Input: part model. Units: mm. Frame: model coordinates. Round coordinates to 2 decimals unless told otherwise and drop trailing zeros. Write each question's results on one line, items separated by ' | '.
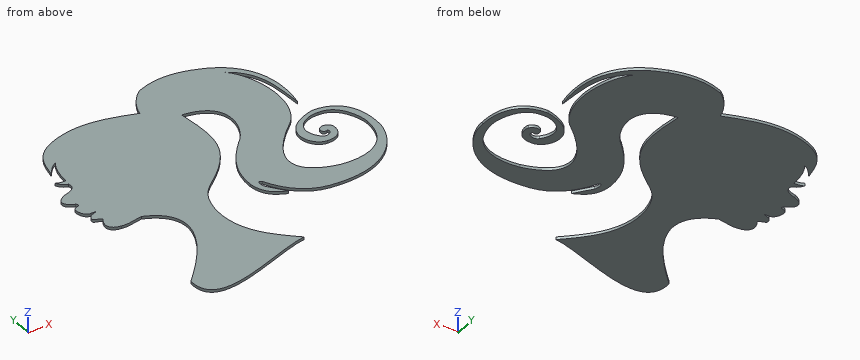
from build123d import *

# Parameters (mm, degrees)
F1_DEPTH = 1


with BuildPart() as f1:
    # F0 (on Top) → F1 (new body)
    with BuildSketch(Plane.XY):
        with BuildLine():
            add(Edge.make_bspline(
                [(-20.8665426716, 18.397650235), (-20.1903553635, 22.148523992), (-18.5927961308, 30.6072682277), (0.8297736088, 36.4578977579), (13.424566628, 32.0204028302), (19.7537988424, 29.7199543566)],
                knots=[0, 0, 0, 0, 0.276946376, 0.6257935478, 1, 1, 1, 1], degree=3))
            add(Edge.make_bspline(
                [(-20.8665426716, 18.397650235), (-19.5796533177, 19.9643534919), (-18.4618644416, 21.7904262245), (-16.4070501924, 22.4652308971)],
                knots=[0, 0, 0, 0, 6.0359163029, 6.0359163029, 6.0359163029, 6.0359163029], degree=3))
            add(Edge.make_bspline(
                [(-19.1014725715, 12.8793083131), (-19.1014725715, 16.4545979351), (-18.215386197, 20.5580331385), (-16.4070501924, 22.4652308971)],
                knots=[0, 0, 0, 0, 9.957400451, 9.957400451, 9.957400451, 9.957400451], degree=3))
            add(Edge.make_bspline(
                [(-22.681472823, 13.5721871629), (-21.7005256563, 12.9922945052), (-20.227715373, 12.7012068406), (-19.1014725715, 12.8793083131)],
                knots=[0, 0, 0, 0, 3.6464342722, 3.6464342722, 3.6464342722, 3.6464342722], degree=3))
            add(Edge.make_bspline(
                [(-19.5205342025, 10.8836535364), (-21.142622456, 11.263910681), (-22.0586042851, 12.5462869182), (-22.681472823, 13.5721871629)],
                knots=[0, 0, 0, 0, 4.1496681824, 4.1496681824, 4.1496681824, 4.1496681824], degree=3))
            add(Edge.make_bspline(
                [(-23.7308889627, 6.6631692462), (-21.9120476395, 7.1236696094), (-18.5412317514, 7.9297339544), (-19.5205342025, 10.8836535364)],
                knots=[0, 0, 0, 0, 5.9615077667, 5.9615077667, 5.9615077667, 5.9615077667], degree=3))
            add(Edge.make_bspline(
                [(-23.7308889627, 0.8257346926), (-26.2068863958, 1.7335914308), (-29.0413927287, 4.5064790174), (-23.7308889627, 6.6631692462)],
                knots=[0, 0, 0, 0, 5.8374345535, 5.8374345535, 5.8374345535, 5.8374345535], degree=3))
            add(Edge.make_bspline(
                [(-23.7308889627, -0.4696604155), (-23.3873687685, -0.4872174759), (-22.8560995311, 0.2822079114), (-23.7308889627, 0.8257346926)],
                knots=[0, 0, 0, 0, 1.2953951082, 1.2953951082, 1.2953951082, 1.2953951082], degree=3))
            add(Edge.make_bspline(
                [(-25.4408102483, -1.531884307), (-25.1299161464, -0.9100947645), (-24.4304016232, -0.5214762059), (-23.7308889627, -0.4696604155)],
                knots=[0, 0, 0, 0, 2.0129953796, 2.0129953796, 2.0129953796, 2.0129953796], degree=3))
            add(Edge.make_bspline(
                [(-22.4216707264, -5.833170151), (-24.9668207233, -6.2141881861), (-25.9071532637, -1.9205028657), (-25.4408102483, -1.531884307)],
                knots=[0, 0, 0, 0, 5.2551178259, 5.2551178259, 5.2551178259, 5.2551178259], degree=3))
            add(Edge.make_bspline(
                [(-20.9138079784, -6.0188561941), (-20.6068530679, -5.7070334442), (-21.582293878, -6.0338505094), (-22.4216707264, -5.833170151)],
                knots=[0, 0, 0, 0, 1.5192528998, 1.5192528998, 1.5192528998, 1.5192528998], degree=3))
            add(Edge.make_bspline(
                [(-23.3263075352, -7.0466995183), (-22.853889813, -6.6050914991), (-21.4558626197, -6.3404192432), (-20.9138079784, -6.0188561941)],
                knots=[0, 0, 0, 0, 2.6223302634, 2.6223302634, 2.6223302634, 2.6223302634], degree=3))
            add(Edge.make_bspline(
                [(-21.2470069528, -10.5123631656), (-21.7241961509, -9.0493401513), (-25.5754273385, -9.9428268093), (-23.3263075352, -7.0466995183)],
                knots=[0, 0, 0, 0, 4.0415733852, 4.0415733852, 4.0415733852, 4.0415733852], degree=3))
            add(Edge.make_bspline(
                [(-18.5455586761, -16.6124049574), (-19.9988428503, -16.5669471025), (-24.3122242391, -15.2729321271), (-21.2470069528, -10.5123631656)],
                knots=[0, 0, 0, 0, 6.6714565616, 6.6714565616, 6.6714565616, 6.6714565616], degree=3))
            add(Edge.make_bspline(
                [(-10.5979545042, -15.9152131528), (-13.2471558948, -16.147610421), (-15.9312561154, -17.2224100679), (-18.5455586761, -16.6124049574)],
                knots=[0, 0, 0, 0, 7.9781256249, 7.9781256249, 7.9781256249, 7.9781256249], degree=3))
            add(Edge.make_bspline(
                [(-17.3396617174, -52.9880858958), (-13.085112907, -48.4555363655), (11.8656428531, -25.2468641847), (-10.5979545042, -15.9152131528)],
                knots=[0, 0, 0, 0, 37.6808772399, 37.6808772399, 37.6808772399, 37.6808772399], degree=3))
            add(Edge.make_bspline(
                [(24.6794633567, -52.9880858958), (12.7007942647, -54.1992671788), (-18.2323064655, -71.822501719), (-17.3396617174, -52.9880858958)],
                knots=[0, 0, 0, 0, 42.0191250741, 42.0191250741, 42.0191250741, 42.0191250741], degree=3))
            add(Edge.make_bspline(
                [(29.9084167928, 21.8148902059), (30.8950484785, 14.8113194584), (32.7630662271, 1.551260361), (20.7029575849, -11.1408703973), (11.5996920553, -16.6471227563), (9.0480540501, -31.2728844387), (14.3939009926, -43.6415991523), (21.2232429507, -49.8474196819), (24.6794633567, -52.9880858958)],
                knots=[0, 0, 0, 0, 0.1970538936, 0.3730877246, 0.5146793148, 0.6758169533, 0.8359361607, 1, 1, 1, 1], degree=3))
            add(Edge.make_bspline(
                [(36.3382212818, 0), (41.4113514125, 4.037628416), (47.6856790483, 19.7234489024), (29.9084167928, 21.8148902059)],
                knots=[0, 0, 0, 0, 22.7427311566, 22.7427311566, 22.7427311566, 22.7427311566], degree=3))
            add(Edge.make_bspline(
                [(26.7475955188, -20.5264855176), (26.4226775616, -11.8059907109), (30.5184200406, -5.9673800133), (36.3382212818, 0)],
                knots=[0, 0, 0, 0, 22.6564937762, 22.6564937762, 22.6564937762, 22.6564937762], degree=3))
            add(Edge.make_bspline(
                [(34.4597883523, -30.0686936826), (31.496912241, -28.7179704756), (27.4011716247, -26.97510086), (26.7475955188, -20.5264855176)],
                knots=[0, 0, 0, 0, 12.2691342385, 12.2691342385, 12.2691342385, 12.2691342385], degree=3))
            add(Edge.make_bspline(
                [(29.987193644, -24.1249073297), (31.4780585468, -26.1061694473), (32.9689234495, -28.0874315649), (34.4597883523, -30.0686936826)],
                knots=[0, 0, 0, 0, 7.4385952728, 7.4385952728, 7.4385952728, 7.4385952728], degree=3))
            add(Edge.make_bspline(
                [(30.6163486093, -21.3921349496), (29.0937069803, -19.5650476962), (29.0937069803, -22.8308942169), (29.987193644, -24.1249073297)],
                knots=[0, 0, 0, 0, 2.8042611954, 2.8042611954, 2.8042611954, 2.8042611954], degree=3))
            add(Edge.make_bspline(
                [(49.8153455555, -35.02195701), (43.0737137794, -34.7288399935), (35.7458516955, -31.9442562759), (30.6163486093, -21.3921349496)],
                knots=[0, 0, 0, 0, 23.545138206, 23.545138206, 23.545138206, 23.545138206], degree=3))
            add(Edge.make_bspline(
                [(77.7483582497, -14.7911049426), (78.2474428415, -21.2455783039), (71.2127014995, -36.9272008538), (49.8153455555, -35.02195701)],
                knots=[0, 0, 0, 0, 34.4897169247, 34.4897169247, 34.4897169247, 34.4897169247], degree=3))
            add(Edge.make_bspline(
                [(64.4583404064, 1.3616352808), (76.0629549623, 0.9637963958), (77.9681950808, -8.9288158342), (77.7483582497, -14.7911049426)],
                knots=[0, 0, 0, 0, 20.9173514336, 20.9173514336, 20.9173514336, 20.9173514336], degree=3))
            add(Edge.make_bspline(
                [(59.4363287091, -14.6286822855), (53.6440759897, -14.4746331498), (48.2831597328, -1.9658291712), (64.4583404064, 1.3616352808)],
                knots=[0, 0, 0, 0, 16.7603955013, 16.7603955013, 16.7603955013, 16.7603955013], degree=3))
            add(Edge.make_bspline(
                [(64.9254620075, -8.5224593058), (65.7523497939, -9.4834351912), (65.8447816968, -15.1524497196), (59.4363287091, -14.6286822855)],
                knots=[0, 0, 0, 0, 8.2107577875, 8.2107577875, 8.2107577875, 8.2107577875], degree=3))
            add(Edge.make_bspline(
                [(60.7119426131, -8.5224593058), (61.0233768821, -7.1668047458), (63.2400512695, -6.5439366736), (64.9254620075, -8.5224593058)],
                knots=[0, 0, 0, 0, 4.2135193944, 4.2135193944, 4.2135193944, 4.2135193944], degree=3))
            add(Edge.make_bspline(
                [(62.4780319631, -9.7865154967), (62.0675943792, -10.4277031496), (60.3455491364, -10.1712280884), (60.7119426131, -8.5224593058)],
                knots=[0, 0, 0, 0, 2.1718447564, 2.1718447564, 2.1718447564, 2.1718447564], degree=3))
            add(Edge.make_bspline(
                [(62.4780319631, -11.3753341138), (62.9469379783, -11.0505707562), (62.8736615181, -10.3177847341), (62.4780319631, -9.7865154967)],
                knots=[0, 0, 0, 0, 1.5888186172, 1.5888186172, 1.5888186172, 1.5888186172], degree=3))
            add(Edge.make_bspline(
                [(58.9657090604, -11.3753341138), (60.144033283, -12.772618793), (61.9759969413, -12.0398327708), (62.4780319631, -11.3753341138)],
                knots=[0, 0, 0, 0, 3.5123229027, 3.5123229027, 3.5123229027, 3.5123229027], degree=3))
            add(Edge.make_bspline(
                [(65.3125420213, -0.5918830284), (60.3213422, 0), (53.2966963947, -4.7204042785), (58.9657090604, -11.3753341138)],
                knots=[0, 0, 0, 0, 12.5125978895, 12.5125978895, 12.5125978895, 12.5125978895], degree=3))
            add(Edge.make_bspline(
                [(75.3649771214, -12.9526508972), (75.2333179116, -8.9721651748), (72.5220516324, -0.4686435277), (65.3125420213, -0.5918830284)],
                knots=[0, 0, 0, 0, 15.9323580724, 15.9323580724, 15.9323580724, 15.9323580724], degree=3))
            add(Edge.make_bspline(
                [(55.5079430342, -27.3152571172), (62.761053443, -28.6342725158), (75.0718563795, -27.3152571172), (75.3649771214, -12.9526508972)],
                knots=[0, 0, 0, 0, 24.5068614916, 24.5068614916, 24.5068614916, 24.5068614916], degree=3))
            add(Edge.make_bspline(
                [(55.5079430342, 0), (37.8463231027, -14.5647795871), (41.0705842078, -23.7978845835), (55.5079430342, -27.3152571172)],
                knots=[0, 0, 0, 0, 27.3152571172, 27.3152571172, 27.3152571172, 27.3152571172], degree=3))
            add(Edge.make_bspline(
                [(53.6933578551, 33.1152714789), (59.9522590637, 27.195526287), (64.3094331026, 9.4182631001), (55.5079430342, 0)],
                knots=[0, 0, 0, 0, 33.1649502411, 33.1649502411, 33.1649502411, 33.1649502411], degree=3))
            add(Edge.make_bspline(
                [(63.429273665, 7.7279442921), (62.56660074, 15.9849859774), (63.7989938259, 26.5835784376), (53.6933578551, 33.1152714789)],
                knots=[0, 0, 0, 0, 27.1901533343, 27.1901533343, 27.1901533343, 27.1901533343], degree=3))
            add(Edge.make_bspline(
                [(45.8327420056, 39.828594774), (49.2567382753, 38.5378040373), (68.2356134057, 32.9920314252), (63.429273665, 7.7279442921)],
                knots=[0, 0, 0, 0, 36.6072354569, 36.6072354569, 36.6072354569, 36.6072354569], degree=3))
            add(Edge.make_bspline(
                [(26.5074167401, 39.828594774), (31.9970119745, 41.9316887856), (37.9454195499, 42.5398573279), (45.8327420056, 39.828594774)],
                knots=[0, 0, 0, 0, 19.3253252655, 19.3253252655, 19.3253252655, 19.3253252655], degree=3))
            add(Edge.make_bspline(
                [(19.7537988424, 29.7199543566), (20.4133884295, 33.497739788), (23.4133824706, 37.7923734486), (26.5074167401, 39.828594774)],
                knots=[0, 0, 0, 0, 12.1571364143, 12.1571364143, 12.1571364143, 12.1571364143], degree=3))
        make_face()
    extrude(amount=F1_DEPTH)


solid = f1.part
1. Contact query for a flat-ended pin moving along its axis: pin 1 (10 mm diameter, centred on x = 30, y = 22.5, fed in from -Z). Output: stop coordinate, or through.
Answer:
pin 1: z = 0
2. Section query A-A, the plane y = 9.5. Count the separate pieces of the cut face and the enclosed holes in it, plus the area to 3 significant figures.
Answer:
separate pieces: 3 | enclosed holes: 0 | area: 69.4 mm^2
3. Line query: line 1 (Y direction, x = 33.5, z = 0.15); line 2 (X direction, y = -2.5, z = 0.8); line 3 (X direction, y = -6, z = 0.35). Output: solid intervals per line, ascending. Write a range as [from, to].
Answer:
line 1: [-29.63, -28.79], [-26.25, -3.09], [21.13, 41.53] | line 2: [-25.51, 27.78], [34.01, 52.62], [56.05, 58.92], [70.69, 73.94] | line 3: [-20.9, 25.18], [31.22, 49.11], [53.94, 56.89], [73.43, 76.22]
